Geometry check sheet. Reference: the model listing, model coordinates, mm. A direction names the side the tool comes from. Coordinates: 2 decimals unless noted, no trailing zeros. Loops run counter-clockwise (first coordinate to the right, second up) from the corner with the lowest first, then second, coordinate; pieces in that order, holes last. Notation, with made-up numbers: (79.25, -11.5) - (95.25, -11.5) arc R28 cw to (95.25, 15.5) - close; hole circle Ø11 at (15, 18.5). An arc over 180 degrees is marked (long way). One line per item, written item: value.
Autodesk Inventor part; units mm, degrees
ref_plane "YZ Plane" through (0, 0, 0) normal (1, 0, 0) x (0, 1, 0)
ref_plane "XZ Plane" through (0, 0, 0) normal (0, 1, 0) x (-1, 0, 0)
ref_plane "XY Plane" through (0, 0, 0) normal (0, 0, 1) x (1, 0, 0)
sketch "Sketch1" plane through (0, 0, 0) normal (1, 0, 0) x (0, 1, 0)
  line L0 (0, 70) -> (-341.3, 70) construction
  line L1 (-341.3, 70) -> (-341.3, 0) construction
  line L2 (-341.3, 0) -> (0, 0)
  line L3 (0, 0) -> (0, 60) construction
  line L4 (0, 70) -> (6, 70)
  line L5 (6, 70) -> (6, 60)
  line L6 (6, 60) -> (0, 60)
  line L7 (0, 50) -> (6, 50)
  line L8 (6, 50) -> (6, 40)
  line L9 (6, 40) -> (0, 40)
  line L10 (0, 30) -> (6, 30)
  line L11 (6, 30) -> (6, 20)
  line L12 (6, 20) -> (0, 20)
  line L13 (0, 10) -> (6, 10)
  line L14 (6, 10) -> (6, 0)
  line L15 (6, 0) -> (0, 0)
  line L16 (0, 60) -> (0, 50)
  line L17 (0, 40) -> (0, 30)
  line L18 (0, 20) -> (0, 10)
  line L19 (-10.15, 28.525) -> (-19.85, 28.525)
  line L20 (-19.85, 28.525) -> (-19.85, 22.675)
  line L21 (-19.85, 22.675) -> (-10.15, 22.675)
  line L22 (-10.15, 22.675) -> (-10.15, 28.525)
  line L23 (-10, 28.6) -> (-331.3, 28.6) construction
  line L24 (-331.3, 28.6) -> (-331.3, 22.6) construction
  line L25 (-331.3, 22.6) -> (-10, 22.6) construction
  line L26 (-10, 22.6) -> (-10, 28.6) construction
  line L27 (-15, 28.6) -> (-15, 22.6) construction
  line L28 (-30.15, 22.675) -> (-30.15, 28.525)
  line L29 (-30.15, 28.525) -> (-39.85, 28.525)
  line L30 (-39.85, 22.675) -> (-30.15, 22.675)
  line L31 (-39.85, 28.525) -> (-39.85, 22.675)
  line L32 (-50.15, 22.675) -> (-50.15, 28.525)
  line L33 (-50.15, 28.525) -> (-59.85, 28.525)
  line L34 (-59.85, 22.675) -> (-50.15, 22.675)
  line L35 (-59.85, 28.525) -> (-59.85, 22.675)
  line L36 (-70.15, 22.675) -> (-70.15, 28.525)
  line L37 (-70.15, 28.525) -> (-79.85, 28.525)
  line L38 (-79.85, 22.675) -> (-70.15, 22.675)
  line L39 (-79.85, 28.525) -> (-79.85, 22.675)
  line L40 (-90.15, 22.675) -> (-90.15, 28.525)
  line L41 (-90.15, 28.525) -> (-99.85, 28.525)
  line L42 (-99.85, 22.675) -> (-90.15, 22.675)
  line L43 (-99.85, 28.525) -> (-99.85, 22.675)
  line L44 (-110.15, 22.675) -> (-110.15, 28.525)
  line L45 (-110.15, 28.525) -> (-119.85, 28.525)
  line L46 (-119.85, 22.675) -> (-110.15, 22.675)
  line L47 (-119.85, 28.525) -> (-119.85, 22.675)
  line L48 (-130.15, 22.675) -> (-130.15, 28.525)
  line L49 (-130.15, 28.525) -> (-139.85, 28.525)
  line L50 (-139.85, 22.675) -> (-130.15, 22.675)
  line L51 (-139.85, 28.525) -> (-139.85, 22.675)
  line L52 (-150.15, 22.675) -> (-150.15, 28.525)
  line L53 (-150.15, 28.525) -> (-159.85, 28.525)
  line L54 (-159.85, 22.675) -> (-150.15, 22.675)
  line L55 (-159.85, 28.525) -> (-159.85, 22.675)
  line L56 (-170.15, 22.675) -> (-170.15, 28.525)
  line L57 (-170.15, 28.525) -> (-179.85, 28.525)
  line L58 (-179.85, 22.675) -> (-170.15, 22.675)
  line L59 (-179.85, 28.525) -> (-179.85, 22.675)
  line L60 (-190.15, 22.675) -> (-190.15, 28.525)
  line L61 (-190.15, 28.525) -> (-199.85, 28.525)
  line L62 (-199.85, 22.675) -> (-190.15, 22.675)
  line L63 (-199.85, 28.525) -> (-199.85, 22.675)
  line L64 (-210.15, 22.675) -> (-210.15, 28.525)
  line L65 (-210.15, 28.525) -> (-219.85, 28.525)
  line L66 (-219.85, 22.675) -> (-210.15, 22.675)
  line L67 (-219.85, 28.525) -> (-219.85, 22.675)
  line L68 (-230.15, 22.675) -> (-230.15, 28.525)
  line L69 (-230.15, 28.525) -> (-239.85, 28.525)
  line L70 (-239.85, 22.675) -> (-230.15, 22.675)
  line L71 (-239.85, 28.525) -> (-239.85, 22.675)
  line L72 (-250.15, 22.675) -> (-250.15, 28.525)
  line L73 (-250.15, 28.525) -> (-259.85, 28.525)
  line L74 (-259.85, 22.675) -> (-250.15, 22.675)
  line L75 (-259.85, 28.525) -> (-259.85, 22.675)
  line L76 (-270.15, 22.675) -> (-270.15, 28.525)
  line L77 (-270.15, 28.525) -> (-279.85, 28.525)
  line L78 (-279.85, 22.675) -> (-270.15, 22.675)
  line L79 (-279.85, 28.525) -> (-279.85, 22.675)
  line L80 (-290.15, 22.675) -> (-290.15, 28.525)
  line L81 (-290.15, 28.525) -> (-299.85, 28.525)
  line L82 (-299.85, 22.675) -> (-290.15, 22.675)
  line L83 (-299.85, 28.525) -> (-299.85, 22.675)
  line L84 (-310.15, 22.675) -> (-310.15, 28.525)
  line L85 (-310.15, 28.525) -> (-319.85, 28.525)
  line L86 (-319.85, 22.675) -> (-310.15, 22.675)
  line L87 (-319.85, 28.525) -> (-319.85, 22.675)
  line L88 (-341.3, 36.1) -> (-256.3, 36.1)
  line L89 (-256.3, 36.1) -> (-256.3, 70)
  line L90 (-341.3, 36.1) -> (-341.3, 0)
  line L91 (-256.3, 70) -> (0, 70)
  point P0 (0, 35)
  point P1 (-170.65, 0)
  point P2 (3, 70)
  point P3 (3, 50)
  point P4 (3, 30)
  point P5 (3, 10)
  point P6 (-10.15, 25.6)
  point P7 (-10, 25.6)
  point P8 (0, 35)
  point P9 (-15, 25.6)
  point P10 (-15, 22.675)
  point P11 (-30.15, 25.6)
  point P12 (-35, 22.675)
  point P13 (-50.15, 25.6)
  point P14 (-55, 22.675)
  point P15 (-70.15, 25.6)
  point P16 (-75, 22.675)
  point P17 (-90.15, 25.6)
  point P18 (-95, 22.675)
  point P19 (-110.15, 25.6)
  point P20 (-115, 22.675)
  point P21 (-130.15, 25.6)
  point P22 (-135, 22.675)
  point P23 (-150.15, 25.6)
  point P24 (-155, 22.675)
  point P25 (-170.15, 25.6)
  point P26 (-175, 22.675)
  point P27 (-190.15, 25.6)
  point P28 (-195, 22.675)
  point P29 (-210.15, 25.6)
  point P30 (-215, 22.675)
  point P31 (-230.15, 25.6)
  point P32 (-235, 22.675)
  point P33 (-250.15, 25.6)
  point P34 (-255, 22.675)
  point P35 (-270.15, 25.6)
  point P36 (-275, 22.675)
  point P37 (-290.15, 25.6)
  point P38 (-295, 22.675)
  point P39 (-310.15, 25.6)
  point P40 (-315, 22.675)
  point P41 (-331.3, 25.6)
  dimension "d7" = 70
  dimension "d18" = 6
  dimension "d21" = 10
  dimension "d24" = 341.3
  dimension "d35" = 20
  dimension "d49" = 5.85
  dimension "d50" = 9.7
  dimension "d51" = 6
  dimension "d52" = 9.4
  dimension "d53" = 10
  dimension "d58" = 10
  dimension "d60" = 5
  dimension "d63" = 20
  dimension "d73" = 10.5
  dimension "d74" = 85
extrude "Extrusion1" add sketch "Sketch1" along normal blind 6
fillet "Fillet1" radius 5 4 edges at (3, -256.3, 70) (3, -256.3, 36.1) (3, -341.3, 36.1) (3, -341.3, 0)
equation "\"d7\" = moduleMountH"
equation "\"d18\" = fingerH"
equation "\"d21\" = fingerW"
equation "\"d24\" = supportL"
equation "\"d35\" = fingerSpacing"
equation "\"d49\" = fingerholeH"
equation "\"d51\" = thickness"
equation "\"d58\" = 0.5 * fingerSpacing"
equation "\"d63\" = fingerSpacing"
equation "\"d74\" = actuatorCableCutoutH"
equation "\"d44\" = thickness"
equation "\"d75\" = supportsFilletR"
equation "\"moduleWidth\" = 118"
equation "\"moduleHeight\" = 96"
equation "\"moduleMountH\" = 70"
equation "\"moduleMountD\" = 6.8"
equation "\"moduleCornerR\" = 5"
equation "\"d4\" = moduleCornerR"
equation "\"d5\" = moduleMountD"
equation "\"d6\" = moduleMountD"
equation "\"d8\" = moduleMountD"
equation "\"d10\" = moduleMountD"
equation "\"moduleOpeningR\" = 25"
equation "\"d13\" = moduleOpeningR"
equation "\"thickness\" = 6"
equation "\"d15\" = thickness"
equation "\"d16\" = 0"
equation "\"kerf\" = 0.15"
equation "\"fingerW\" = 10"
equation "\"fingerSpacing\" = 20"
equation "\"fingerholeW\" = fingerW - 2 * kerf"
equation "\"fingerholeH\" = thickness - kerf"
equation "\"moduleMountClearance\" = 19"
equation "\"actuatorW\" = 28"
equation "\"actuatorH\" = 40.8"
equation "\"openingMFC\" = 45"
equation "\"d28\" = thickness"
equation "\"d29\" = thickness"
equation "\"d30\" = 0.5 * actuatorH + thickness"
equation "\"d31\" = 15"
equation "\"d32\" = fingerholeH"
equation "\"d33\" = fingerholeW"
equation "\"d41\" = fingerholeH"
equation "\"d42\" = fingerholeW"
equation "\"chairThickness\" = 12.7"
equation "\"supportL\" = -chairThickness + dildoL + actuatorMountL - thickness"
equation "\"d0\" = moduleHeight"
equation "\"d1\" = moduleWidth"
equation "\"d17\" = openingMFC"
equation "\"d19\" = moduleMountClearance"
equation "\"fingerH\" = thickness"
equation "\"supportSpacingFromMounting\" = 15"
equation "\"d54\" = fingerholeH"
equation "\"d55\" = fingerholeW"
equation "\"d64\" = 9.4"
equation "\"supportsCTCZ\" = d64"
equation "\"supportXW\" = -2 * thickness + moduleMountW - 2 * supportSpacingFromMounting + kerf"
equation "\"actuatorCableW\" = 35"
equation "\"actuatorCableCutoutH\" = 85"
equation "\"supportsFilletR\" = 5"
properties part number "Module_supportZ_cableNotch_MFC"
(1) Cross-section at C-C on z = 45.5. Record the cut outline in (x, y), and give its area (3 significant figures).
Reply:
outline: (0, -256.3) - (6, -256.3) - (6, 6) - (0, 6) - close
area: 1,570 mm2
(2) Release check for a two-part mould opening along Y. For faces 4 (the face through (3, -275, 22.675)), 5 (the face through (3, -310.15, 26)), 6 (the face through (3, 0, 35)), 7 (the face through (3, -163, 0)) record: pulls with the +Y half, pulls with the -Y half, needs draft (parallel to the pull), parting line crosses it, or undercut.
Reply:
face 4: undercut
face 5: undercut
face 6: pulls with the +Y half
face 7: needs draft
(3) Cross-section at B-B on x = 5.1. State how many separate pieces and enclosed holes the cut face has, and give its area (3 significant figures).
Reply:
separate pieces: 1
enclosed holes: 16
area: 20,300 mm2
(4) Material ranges on probe 1 along Z at (x, y) = (3.7, -15) (3 decimals); probe 2 along Z at (x, y) = (1.25, -288.5); probe 3 along Y at (x, z) = (2.2, 16.5), recorded low to high. Write a range as from..to.
Reply:
probe 1: 0..22.675, 28.525..70
probe 2: 0..36.1
probe 3: -341.3..0
(5) Access from +Z, -Z, +X, -X, +Y, -Y to the whole of each face (thin tool, end or side, straight path). Record for faces 1 (the face through (3, 3, 50)), 2 (the face through (3, 6, 25)), 3 (the face through (3, -319.85, 26)).
Reply:
face 1: +X, -X, +Y
face 2: +Z, -Z, +X, -X, +Y
face 3: +X, -X
(6) Cross-section at A-A on y = -174. Record the cut outline in (x, z) (3 decimals).
Reply:
outline: (0, 0) - (6, 0) - (6, 22.675) - (0, 22.675) - close; (0, 28.525) - (6, 28.525) - (6, 70) - (0, 70) - close
(7) Go/stop test with flat-tipped pins: pin 1 Ø1.8 at (x, y) = (4.5, -273.5) entering from +Z; pin 2 Ø1.5 at (x, z) = (1, 59.5) entering from -Y; pin 3 Ø3 at (x, z) = (4, 35.5) entering from +Y. Record where each tip stops, or that it passes through.
Reply:
pin 1: z = 36.1
pin 2: y = -256.3
pin 3: y = 0
